Autodesk Inventor part; units mm, degrees
ref_plane "YZ Plane" through (0, 0, 0) normal (1, 0, 0) x (0, 1, 0)
ref_plane "XZ Plane" through (0, 0, 0) normal (0, 1, 0) x (-1, 0, 0)
ref_plane "XY Plane" through (0, 0, 0) normal (0, 0, 1) x (1, 0, 0)
sketch "スケッチ2" plane through (0, 0, 0) normal (1, 0, 0) x (0, 1, 0)
  line L0 (0, 0) -> (-59.3543, 0)
  line L1 (-59.3543, -20) -> (1.7498, -20)
  line L2 (0, 0) -> (58.4526, 10.3068)
  line L3 (61.9255, -9.3894) -> (1.7498, -20)
  arc A0 (62.5368, 10.1792) -> (58.4526, 10.3068) centre (60.1891, 0.4587) ccw
  arc A1 (61.9255, -9.3894) -> (65.7198, -7.8726) centre (60.1891, 0.4587) ccw
  arc A2 (-63.3543, -19.1652) -> (-59.3543, -20) centre (-59.3543, -10) ccw
  arc A3 (-59.3543, 0) -> (-63.3543, -0.8348) centre (-59.3543, -10) ccw
  arc A4 (-59.3543, -14) -> (-59.3543, -6) centre (-59.3543, -10) ccw
  line L4 (-59.3543, -6) -> (-63.3543, -6)
  line L5 (-59.3543, -14) -> (-63.3543, -14)
  line L6 (-63.3543, -0.8348) -> (-63.3543, -6)
  line L7 (-63.3543, -14) -> (-63.3543, -19.1652)
  line L8 (65.7198, -7.8726) -> (65.3114, -5.5567)
  line L9 (62.9451, 7.8632) -> (62.5368, 10.1792)
  line L10 (1.7498, -20) -> (0, 0)
  line L11 (65.3114, -5.5567) -> (62.9451, 7.8632)
  dimension "d21" = 20
  dimension "d22" = 10
  dimension "d23" = 170
  dimension "d27" = 10
  dimension "d31" = 8
  dimension "d33" = 4
  dimension "d35" = 4
  dimension "d36" = 120
  dimension "d139" = 20
extrude "押し出し1" add sketch "スケッチ2" along normal blind 2
sketch "スケッチ4" plane through (0, 0, 0) normal (-1, 0, 0) x (0, 0, 1)
  line L0 (-20, 1.7498) -> (-9.3894, 61.9255)
  line L1 (-20, -59.3543) -> (-20, 1.7498)
  circle A0 centre (-17, -18.5891) radius 1
  circle A1 centre (-13.5138, 21.2587) radius 1
  line L2 (-17, -18.5891) -> (-13.5138, 21.2587)
  line L3 (-20, 1.7498) -> (0, 0)
  dimension "d57" = 2
  dimension "d59" = 40
  dimension "d60" = 175
  dimension "d61" = 3
  dimension "d62" = 3
hole "穴2" at (0, -18.5891, -17) at (0, 21.2587, -13.5138) direction (1, 0, 0) diameter 1.6 end through all
sketch "スケッチ6" plane through (2, 0, 0) normal (1, 0, 0) x (0, 0, -1)
  line L0 (20, 1.7498) -> (9.3894, 61.9255)
  arc A0 (9.3894, 61.9255) -> (7.8726, 65.7198) centre (-0.4587, 60.1891) ccw
  line L1 (7.8726, 65.7198) -> (-10.1792, 62.5368)
  arc A1 (-10.1792, 62.5368) -> (-10.3068, 58.4526) centre (-0.4587, 60.1891) ccw
  line L2 (-10.3068, 58.4526) -> (0, 0)
  line L3 (-5.04, 28.5832) -> (-8.2539, 32.4135)
  line L4 (-10.1792, 62.5368) -> (-13.4634, 61.9577)
  line L5 (-13.4634, 61.9577) -> (-8.2539, 32.4135)
  line L6 (7.8726, 65.7198) -> (11.1568, 66.2989)
  line L7 (11.1568, 66.2989) -> (16.3663, 36.7547)
  line L8 (16.3663, 36.7547) -> (14.6562, 32.0562)
  dimension "d75" = 150
  dimension "d76" = 150
  dimension "d77" = 2.5
  dimension "d78" = 2.5
  dimension "d79" = 30
extrude "押し出し2" add sketch "スケッチ6" against normal blind 2
sketch "スケッチ5" plane through (2, 0, 0) normal (1, 0, 0) x (0, 0, -1)
  line L0 (7.8726, 65.7198) -> (-10.1792, 62.5368)
  circle A0 centre (-8.1635, 57.8151) radius 1.5
  circle A1 centre (7.5934, 60.5934) radius 1.5
  line L1 (14.6562, 32.0562) -> (20, 1.7498)
  line L2 (20, 1.7498) -> (20, -59.3543)
  arc A2 (19.1652, -63.3543) -> (20, -59.3543) centre (10, -59.3543) ccw
  line L3 (19.1652, -63.3543) -> (14, -63.3543)
  line L4 (14, -63.3543) -> (14, -59.3543)
  arc A3 (14, -59.3543) -> (6, -59.3543) centre (10, -59.3543) ccw
  line L5 (6, -59.3543) -> (6, -63.3543)
  line L6 (6, -63.3543) -> (0.8348, -63.3543)
  arc A4 (0, -59.3543) -> (0.8348, -63.3543) centre (10, -59.3543) ccw
  line L7 (0, -59.3543) -> (0, 0)
  line L8 (0, 0) -> (-5.04, 28.5832)
  circle A5 centre (17, -18.5891) radius 0.8
  circle A6 centre (13.5138, 21.2587) radius 0.8
  line L9 (-8.2539, 32.4135) -> (-13.4634, 61.9577)
  line L10 (-13.4634, 61.9577) -> (11.1568, 66.2989)
  line L11 (11.1568, 66.2989) -> (16.3663, 36.7547)
  line L12 (16.3663, 36.7547) -> (14.6562, 32.0562)
  line L13 (-5.04, 28.5832) -> (-8.2539, 32.4135)
  point P0 (3.5148, 90.434)
  point P1 (-14.537, 87.251)
  point P2 (-10.1792, 62.5368)
  dimension "d72" = 3
  dimension "d114" = 16
  dimension "d174" = 5
  dimension "d175" = 5
  dimension "d176" = 4.5
hole "穴3" at (2, 57.8151, 8.1635) at (2, 60.5934, -7.5934) direction (-1, 0, 0) diameter 4 end through all
sketch "スケッチ7" plane through (2, 0, 0) normal (1, 0, 0) x (0, 0, -1)
  arc A0 (0, -59.3543) -> (0.8348, -63.3543) centre (10, -59.3543) ccw
  line L0 (0.8348, -63.3543) -> (6, -63.3543)
  circle A1 centre (3, -59.3543) radius 1
  dimension "d89" = 4
  dimension "d90" = 7
  dimension "d91" = 2
hole "穴4" at (2, -59.3543, -3) direction (-1, 0, 0) diameter 2 end through all
pattern_circular "円形状パターン3" count 5 over 180 about axis through (0, -59.3543, -10) along (-1, 0, 0) of "穴4"
sketch "スケッチ8" plane through (2, 0, 0) normal (1, 0, 0) x (0, 0, -1)
  line L0 (11.1568, 66.2989) -> (-13.4634, 61.9577)
  line L1 (-13.4634, 61.9577) -> (-8.2539, 32.4135)
  circle A0 centre (-7.1216, 51.9062) radius 1.5
  circle A1 centre (8.6353, 54.6846) radius 1.5
  point P0 (7.8726, 65.7198)
  point P1 (-10.1792, 62.5368)
  dimension "d102" = 11
  dimension "d103" = 11
  dimension "d104" = 16
  dimension "d105" = 4.5
  dimension "d106" = 3
hole "穴5" at (2, 51.9062, 7.1216) at (2, 54.6846, -8.6353) direction (-1, 0, 0) diameter 3.5 end through all
sketch "スケッチ11" plane through (2, 0, 0) normal (1, 0, 0) x (0, 0, -1)
  circle A0 centre (-7.1216, 51.9062) radius 1.75
  circle A1 centre (8.6353, 54.6846) radius 1.75
  line L0 (-13.4634, 61.9577) -> (-8.2539, 32.4135)
  circle A2 centre (-4.5169, 37.1341) radius 1.5
  circle A3 centre (11.24, 39.9125) radius 1.5
  dimension "d124" = 3
  dimension "d126" = 16
  dimension "d127" = 15
  dimension "d128" = 4.5
  dimension "d130" = 15
hole "穴6" at (2, 37.1341, 4.5169) at (2, 39.9125, -11.24) direction (-1, 0, 0) diameter 3.5 end through all
sketch "スケッチ13" plane through (2, 0, 0) normal (1, 0, 0) x (0, 0, -1)
  line L0 (0, 0) -> (0, -59.3543)
  line L1 (20, -59.3543) -> (20, 1.7498)
  line L2 (20, 1.7498) -> (14.6562, 32.0562)
  line L3 (11.1568, 66.2989) -> (-13.4634, 61.9577)
  line L4 (-5.04, 28.5832) -> (0, 0)
  line L5 (-0.4338, 31.2538) -> (10.7167, 25.6042)
  line L6 (10.7167, 25.6042) -> (2.171, 16.4817)
  line L7 (2.171, 16.4817) -> (-0.4338, 31.2538)
  line L8 (4.2547, 4.664) -> (12.8005, 13.7865)
  line L9 (12.8005, 13.7865) -> (15.4052, -0.9856)
  line L10 (15.4052, -0.9856) -> (4.2547, 4.664)
  line L11 (5, -5.4856) -> (15, -12.9856)
  line L12 (5, -20.4856) -> (5, -5.4856)
  line L13 (15, -12.9856) -> (5, -20.4856)
  line L14 (5, -32.4856) -> (15, -24.9856)
  line L15 (15, -24.9856) -> (15, -39.9856)
  line L16 (15, -39.9856) -> (5, -32.4856)
  point P0 (9.3894, 61.9255)
  point P1 (7.8726, 65.7198)
  point P2 (-10.1792, 62.5368)
  point P3 (-10.3068, 58.4526)
  dimension "d147" = 5
  dimension "d149" = 5
  dimension "d160" = 5
  dimension "d162" = 40
  dimension "d163" = 52
  dimension "d164" = 12
  dimension "d166" = 5
  dimension "d177" = 10
  dimension "d178" = 15
  dimension "d179" = 12
extrude "押し出し5" cut sketch "スケッチ13" against normal blind 2
fillet "フィレット2" radius 2 12 edges at (1, -24.9856, -15) (1, 13.7865, -12.8005) (1, 31.2538, 0.4338) (1, -5.4856, -5) (1, 4.664, -4.2547) (1, -32.4856, -5) (1, 25.6042, -10.7167) (1, -12.9856, -15) (1, -0.9856, -15.4052) (1, -39.9856, -15) (1, -20.4856, -5) (1, 16.4817, -2.171)
properties part number "Arm_Link_1" material "アルミニウム 6061"
Can you work these out from the model? Positions are in its coordinate system, mm. A direction names the side the tool comes from. Give positions to 0.01 mm unless a question says otherwise; leave off trailing zeros. Loops run counter-clockwise (first coordinate to the right, second up) from the corner with the lowest first, then second, coordinate; pieces in that order, holes last. Notation, with made-up numbers: (89, -31.75) -> (136, -31.75) arc R33 cw to (136, 2.25) -> close; hole circle Ø11 at (28.25, 68). An arc over 180 degrees is marked (long way). Use one line per item in the form item = value.
1) For faces 4 (the face through (2, 15, -7)), 5 (the face through (1.01, 21.56, -6.93)), which set-ups out of +Z, -Z, +X, -X, +Y, -Y let a thin tool reach every point of the face, with its end or its side?
Answers:
face_4 = +Z, -Z, +X, +Y, -Y
face_5 = +X, -X
2) If we section it at A-A (x = 0.3): Count the separate pieces of the cut face and the enclosed holes in it, plus the area to 3 significant figures.
Answers:
separate_pieces = 1
enclosed_holes = 17
area = 2,320 mm²
3) We'd pull the mould along Z, two halves only. Please class faces 1 (the face through (0.99, 17.12, -17.29)), 2 (the face through (0, 15, -7)), 3 (the face through (0.99, 39.39, -12.91)): released by +Z, released by -Z, zero draft, split by the parting line, or undercut.
Answers:
face_1 = released by -Z
face_2 = zero draft
face_3 = undercut
4) If we section it at B-B (y = -49.5): Please give me the cut outline in (x, z).
Answers:
outline = (0, -20) -> (2, -20) -> (2, 0) -> (0, 0) -> close
5) I need wall thicknesses on line 1 along Y through (x, z) = (1.7, 7); line 2 along Z through (x, y) = (0.65, 59.5); line 3 along Z through (x, y) = (0.8, -37). Which ranges of each line are inside material? Lowest first, please.
Answers:
line_1 = 30.92 to 50.16, 53.65 to 56.19, 59.44 to 63.1
line_2 = -12.36 to -9.27, -5.92 to 7.09, 9.24 to 13.03
line_3 = -20 to -14.72, -11.02 to 0
6) Will these pins go through, and if not, where does the flat tip stop? pin 1 (1.5 mm diameter, centred on y = -31.5, z = -8, fed in from -X); pin 2 (1 mm diameter, centred on x = 2, z = -10.5, fed in from +Y).
Answers:
pin_1 = through
pin_2 = 66.27
